Can you work these out from the model? Positions are in its coordinate system, mm. A direction names the side the tool comes from. Give positions to 0.01 mm unless a question says otherwise; leave off trailing zeros. Order: outer loops, then holes, each group sorted by start corner. A loop starts at its lowest first (then second) coordinate and runs counter-clockwise, first axis right, second up. Notation, with made-up numbers: (38, 81.25) - (56, 81.25) arc R18 ccw to (56, 114.25) - close; hole circle Ø7 at (-20.5, -39). An arc over 180 degrees is marked (long way). Answer as a JSON object with one key per item and string values.
Autodesk Inventor part; units mm, degrees
ref_plane "YZ Plane" through (0, 0, 0) normal (1, 0, 0) x (0, 1, 0)
ref_plane "XZ Plane" through (0, 0, 0) normal (0, 1, 0) x (-1, 0, 0)
ref_plane "XY Plane" through (0, 0, 0) normal (0, 0, 1) x (1, 0, 0)
sketch "Sketch1" plane through (0, 0, 0) normal (0, 0, 1) x (1, 0, 0)
  circle A0 centre (0, 0) radius 27.5
  dimension "d0" = 55
extrude "Extrusion1" add sketch "Sketch1" along normal blind 25
sketch "Sketch2" plane through (0, 0, 0) normal (0, 0, -1) x (-1, 0, 0)
  line L0 (6.1, -11.3) -> (-6.1, -11.3)
  line L1 (-6.1, -11.3) -> (-6.1, 11.3)
  line L2 (-6.1, 11.3) -> (6.1, 11.3)
  line L3 (6.1, 11.3) -> (6.1, -11.3)
  circle A0 centre (0, 0) radius 27.5
  dimension "d4" = 12.2
  dimension "d5" = 55
  dimension "d6" = 22.6
  dimension "d7" = 6.1
  dimension "d8" = 11.3
extrude "Extrusion2" cut sketch "Sketch2" against normal blind 23 contours L0 L1 L2 L3
sketch "Sketch3" plane through (0, 0, 0) normal (0, 0, -1) x (-1, 0, 0)
  line L0 (-6.1, 11.3) -> (6.1, 11.3)
  line L1 (6.1, -11.3) -> (-6.1, -11.3)
  line L2 (6.1, 11.3) -> (6.1, -11.3)
  line L3 (-6.1, -11.3) -> (-6.1, 11.3)
  line L4 (6.1, -16.5) -> (-6.1, -16.5)
  line L5 (-6.1, -16.5) -> (-6.1, 16.5)
  line L6 (-6.1, 16.5) -> (6.1, 16.5)
  line L7 (6.1, 16.5) -> (6.1, -16.5)
  point P0 (0, 0)
  dimension "d11" = 22.6
  dimension "d12" = 12.2
  dimension "d13" = 5.2
  dimension "d14" = 5.2
extrude "Extrusion3" cut sketch "Sketch3" against normal blind 6 contours L5 L6 L7 L0 | L1 L7 L4 L5
sketch "Sketch4" plane through (0, 0, 0) normal (0, 0, -1) x (-1, 0, 0)
  line L0 (-6.1, -16.5) -> (-6.1, 16.5)
  line L1 (6.1, 16.5) -> (6.1, -16.5)
  line L2 (-6.1, 16.5) -> (6.1, 16.5)
  line L3 (6.1, -16.5) -> (-6.1, -16.5)
  line L4 (6.1, 11.3) -> (-6.1, 11.3)
  line L5 (-6.1, -11.3) -> (6.1, -11.3)
  line L6 (-6.1, 16.5) -> (6.1, 16.5)
  line L7 (2, 16.5) -> (2, 27.4272)
  circle A0 centre (0, 0) radius 27.5
  line L8 (-2, 16.5) -> (-2, 27.4272)
  arc A1 (2, 27.4272) -> (-2, 27.4272) centre (0, 0) ccw
  line L9 (2, 16.5) -> (2, 11.3)
  line L10 (-2, 16.5) -> (-2, 11.3)
  dimension "d17" = 12.2
  dimension "d18" = 33
  dimension "d19" = 22.6
  dimension "d20" = 4
  dimension "d21" = 4.1
extrude "Extrusion4" cut sketch "Sketch4" against normal blind 18 contours L10 L2 L9 L4 | L8 A0 L7 L2
hole "Hole2" at (21.1, -0.2, 0) direction (0, 0, 1) diameter 1.567 depth 4.2 tip angle 118
hole "Hole3" at (-21.1, -0.2, 0) direction (0, 0, 1) diameter 1.567 depth 4.2 tip angle 118
properties part number "speaker_base"
Q1. I'm going to push flat-ended pins straight in: pin 1 Ø3.5 at (x, z) = (-2, 10.5) entering from +Y; pin 2 Ø3 at (x, z) = (0.5, 20) entering from +Y; pin 3 Ø5 at (y, z) = (19, 18) entering from +X; pin 4 Ø3.5 at (x, y) = (4.5, 14.5) entering from -Z. Where does each tip first touch, or does it pass through?
Recorded:
{"pin 1": "stops at y = 27.43", "pin 2": "stops at y = 27.5", "pin 3": "stops at x = 22", "pin 4": "stops at z = 0"}
Q2. We'd pull the mould along X, two halves only. Please class faces 1 (the face through (-4, 14, 6)), 2 (the face through (-6.5, 0.3, 0)), 3 (the face through (-5.961, 26.846, 12.325)): released by +X, released by -X, zero draft, split by the parting line, or undercut.
Recorded:
{"face 1": "undercut", "face 2": "zero draft", "face 3": "split by the parting line"}
Q3. If we section it at D-D, the plane z = 13: Please give me the cut outline in (x, y).
Recorded:
{"outline": "(-6.1, -11.3) - (-6.1, 11.3) - (-2, 11.3) - (-2, 27.43) arc R27.5 ccw (long way) to (2, 27.43) - (2, 11.3) - (6.1, 11.3) - (6.1, -11.3) - close"}
Q4. If we section it at B-B, the plane z = 3: Please give me the cut outline in (x, y).
Recorded:
{"outline": "(-6.1, -16.5) - (-6.1, 16.5) - (-2, 16.5) - (-2, 27.43) arc R27.5 ccw (long way) to (2, 27.43) - (2, 16.5) - (6.1, 16.5) - (6.1, -16.5) - close; hole circle Ø1.57 at (-21.1, -0.2); hole circle Ø1.57 at (21.1, -0.2)"}
Q5. I need wall thicknesses on L1, parallel to X at y = -0.2, z = 2.7; L2, parallel to X at y = -8.5, z = 6.75; L3, parallel to Z at x = 4, y = -13.5. Which ranges of each line are inside material? Lowest first, please.
Recorded:
{"L1": "x = -27.5 to -21.88, -20.32 to -6.1, 6.1 to 20.32, 21.88 to 27.5", "L2": "x = -26.15 to -6.1, 6.1 to 26.15", "L3": "z = 6 to 25"}
Q6. If we section it at C-C, the plane x = 4.5: Please give me the cut outline in (y, z).
Recorded:
{"outline": "(-27.13, 0) - (-16.5, 0) - (-16.5, 6) - (-11.3, 6) - (-11.3, 23) - (11.3, 23) - (11.3, 6) - (16.5, 6) - (16.5, 0) - (27.13, 0) - (27.13, 25) - (-27.13, 25) - close"}
Q7. If we section it at A-A, the plane y = 23.5: Please give me the cut outline in (x, z).
Recorded:
{"outline": "(-14.28, 0) - (-2, 0) - (-2, 18) - (2, 18) - (2, 0) - (14.28, 0) - (14.28, 25) - (-14.28, 25) - close"}
Q8. Which directions (+Z, -Z, +X, -X, +Y, -Y) give clear straight access to the entire face, cutting with the end or side of a thin tool? Please do faces 4 (the face through (2, 19, 9)), 5 (the face through (-6.1, 0, 11)), 6 (the face through (0, 0, 25)).
Recorded:
{"face 4": "-Z, +Y", "face 5": "-Z", "face 6": "+Z, +X, -X, +Y, -Y"}
